Here's how the part is built. I have some questions about the finished solid (model axes, mm). A direction names the side the tool comes from. Round coordinates to 2 decimals unless told otherwise and drop trailing zeros. Order: outer loops, then holes, each group sorted by start corner. A loop starts at its lowest first (then second) coordinate and runs counter-clockwise, first axis right, second up.
```python
from build123d import *

# Parameters (mm, degrees)
SKETCH1_R           = 14.605
SKETCH1_R_2         = 12.7
BOSS_EXTRUDE1_DEPTH = 25.4
FILLET1_R           = 1.27
SKETCH3_R           = 12.7
BOSS_EXTRUDE2_DEPTH = 1.27


with BuildPart() as part:
    # Sketch1 → Boss-Extrude1 (new body)
    with BuildSketch(Plane(origin=(0, 0, 0), x_dir=(0, 0, -1), z_dir=(1, 0, 0))):
        Circle(SKETCH1_R)
        Circle(SKETCH1_R_2, mode=Mode.SUBTRACT)
    extrude(amount=BOSS_EXTRUDE1_DEPTH)

    # Fillet1
    fillet1_edges = [part.edges().sort_by_distance(p)[0] for p in [
        (25.4, 0, 14.605),
    ]]
    fillet(fillet1_edges, radius=FILLET1_R)

    # Sketch3 → Boss-Extrude2 (add)
    with BuildSketch(Plane(origin=(25.4, 0, 0), x_dir=(0, 0, -1), z_dir=(1, 0, 0))):
        Circle(SKETCH3_R)
    extrude(amount=-BOSS_EXTRUDE2_DEPTH)


solid = part.part
```
1. I'm going to push flat-ended pins straight in: P1, Ø7.5, axis at y = 6, z = 4, coming from the -X side; P2, Ø1.5, axis at x = 13.5, z = 4, coming from the -Y side; P3, Ø12, axis at x = 4.5, y = 10, coming from the +Z side. Where does each tip first touch, or does it pass through?
Evaluation:
P1: stops at x = 24.13
P2: stops at y = -14.24
P3: stops at z = 14.05
2. If we section it at A-A, the plane y = 0: Write out the boundary of the cut face in (x, z) (3 decimals).
Evaluation:
outline: (0, -14.605) - (24.13, -14.605) arc R1.27 ccw to (25.4, -13.335) - (25.4, 13.335) arc R1.27 ccw to (24.13, 14.605) - (0, 14.605) - (0, 12.7) - (24.13, 12.7) - (24.13, -12.7) - (0, -12.7) - close
3. On a 3-axis mill with a long thin cutter (end or side, diameter ignored), from which of +Z, -Z, +X, -X, +Y, -Y can I reach the whole of each face in a straight line? I mean faces 1 (the flat face through (25.4, 0, 0)), 2 (the cylindrical face through (11.9, -12.4, 2.75)). Say none if no direction works.
Evaluation:
face 1: +Z, -Z, +X, +Y, -Y
face 2: -X
4. If we mould it in two halves opening along Z, with no side actions, what happens to faces 3 (the cylindrical face through (11.896, 9.871, 10.764)), 4 (the flat face through (0, 7, 11)), 5 (the flat face through (24.13, 0, 0))? For each: released by +Z, released by -Z, zero draft, split by the parting line, or undercut.
Evaluation:
face 3: split by the parting line
face 4: zero draft
face 5: undercut
5. I need wall thicknesses on probe 1 along Y at (x, z) = (6.5, 0) (3 decimals); probe 2 along X at (y, z) = (-6, -4.5); probe 3 along Z at (x, y) = (4.75, -9.5). Which ranges of each line are inside material? Lowest first, please.
Evaluation:
probe 1: y = -14.605 to -12.7, 12.7 to 14.605
probe 2: x = 24.13 to 25.4
probe 3: z = -11.09 to -8.43, 8.43 to 11.09
6. If we section it at C-C, the plane x = 16.5: Write out the boundary of the cut face in (y, z) (3 decimals), and give its area (3 significant figures).
Evaluation:
outline: circle Ø29.21 at (0, 0); hole circle Ø25.4 at (0, 0)
area: 163 mm2
